```python
from build123d import *

# Parameters (mm, degrees)
SKETCH1_W           = 133.35
SKETCH1_H           = 38.1
BOSS_EXTRUDE1_DEPTH = 12.7
SKETCH2_R           = 3.175
CUT_EXTRUDE1_DEPTH  = 111.707422131
CAVITY1_DEPTH       = 12.7
CUT_EXTRUDE2_DEPTH  = 108.192417986
CUT_EXTRUDE4_DEPTH  = 108.192417986
CUT_EXTRUDE6_DEPTH  = 108.000606538
CUT_EXTRUDE7_DEPTH  = 105.814568341


# Read off the part's stored shape, not the designer's step: Cavity1
with BuildPart() as part:
    # Sketch1 → Boss-Extrude1 (new body)
    with BuildSketch(Plane.XY):
        with Locations((36.491047297, -7.135705236)):
            Rectangle(SKETCH1_W, SKETCH1_H)
    extrude(amount=BOSS_EXTRUDE1_DEPTH)

    # Sketch2 → Cut-Extrude1 (cut, through all)
    with BuildSketch(Plane(origin=(0, 11.914294764, 0), x_dir=(1, 0, 0), z_dir=(0, 1, 0))):
        with Locations(Location((-22.563952703, -6.35, 0), (0, 0, 270))):
            Circle(SKETCH2_R)
        with Locations(Location((25.188047297, -6.35, 0), (0, 0, 270))):
            Circle(SKETCH2_R)
    extrude(amount=-CUT_EXTRUDE1_DEPTH, mode=Mode.SUBTRACT)

    # Cavity1 outline → Cavity1 (cut)
    with BuildSketch(Plane.XY):
        with BuildLine():
            Line((96.096303093, 11.914294764), (94.056580093, 11.914294764))
            ThreePointArc((94.056580093, 11.914294764), (90.695637122, -2.438784083), (103.166047297, -10.299806924))
            Line((103.166047297, -10.299806924), (103.166047297, -9.052983376))
            ThreePointArc((103.166047297, -9.052983376), (91.591067883, -1.280306677), (96.096303093, 11.914294764))
        make_face()
    extrude(amount=CAVITY1_DEPTH, mode=Mode.SUBTRACT)

    # Sketch4 → Cut-Extrude2 (cut, through all)
    with BuildSketch(Plane(origin=(0, 0, 0), x_dir=(-1, 0, 0), z_dir=(0, 0, -1))):
        Polygon((-103.836015624, 12.337344095), (-103.707966328, -9.632256534), (-101.439664514, -9.485914481), (-98.220139359, -8.863960758), (-94.579880804, -6.924928563), (-91.031086031, -2.168811857), (-90.317668525, 2.879988954), (-91.085877767, 6.8566015), (-93.116460279, 9.831236447), (-96.207936138, 13.398323976), align=None)
    extrude(amount=-CUT_EXTRUDE2_DEPTH, mode=Mode.SUBTRACT)

    # Sketch9 → Cut-Extrude4 (cut, through all)
    with BuildSketch(Plane.XY.offset(12.7)):
        Polygon((-30.183952703, -13.474806924), (119.048045807, -13.474806924), (119.048045807, -32.591302601), (-30.183952703, -32.591302601), (-44.866857433, -32.591302601), (-44.866857433, 12.516766533), (-30.183952703, 12.516766533), align=None)
    extrude(amount=-CUT_EXTRUDE4_DEPTH, mode=Mode.SUBTRACT)

    # Sketch11 → Cut-Extrude6 (cut, through all)
    with BuildSketch(Plane(origin=(0, 11.914294764, 0), x_dir=(1, 0, 0), z_dir=(0, 1, 0))):
        with BuildLine():
            Line((-22.563952703, 0), (-30.183952703, 0))
            Line((-30.183952703, 0), (-30.183952703, -12.7))
            Line((-30.183952703, -12.7), (-22.563952703, -12.7))
            ThreePointArc((-22.563952703, -12.7), (-28.913952703, -6.35), (-22.563952703, 0))
        make_face()
    extrude(amount=-CUT_EXTRUDE6_DEPTH, mode=Mode.SUBTRACT)

    # Sketch12 → Cut-Extrude7 (cut, through all)
    with BuildSketch(Plane.XY):
        with BuildLine():
            Line((34.840047297, 8.739294764), (47.329311848, 8.739294764))
            ThreePointArc((47.329311848, 8.739294764), (63.205042995, 7.678873093), (78.798708551, 4.516448692))
            ThreePointArc((78.798708551, 4.516448692), (84.297585987, 1.423684462), (87.687974389, -3.896852177))
            Line((87.687974389, -3.896852177), (87.782466122, -4.180292862))
            ThreePointArc((87.782466122, -4.180292862), (87.135514906, -8.32519055), (83.381577499, -10.197802807))
            Line((83.381577499, -10.197802807), (46.450888554, -9.684330956))
            ThreePointArc((46.450888554, -9.684330956), (35.893420387, -5.181749435), (31.538047297, 5.437294764))
            ThreePointArc((31.538047297, 5.437294764), (32.505180706, 7.772161355), (34.840047297, 8.739294764))
        make_face()
        with BuildLine():
            Line((18.838047297, 5.437294764), (18.838047297, -6.997806924))
            ThreePointArc((18.838047297, -6.997806924), (17.870913889, -9.332673515), (15.536047297, -10.299806924))
            Line((15.536047297, -10.299806924), (-12.911952703, -10.299806924))
            ThreePointArc((-12.911952703, -10.299806924), (-15.246819294, -9.332673515), (-16.213952703, -6.997806924))
            Line((-16.213952703, -6.997806924), (-16.213952703, 5.437294764))
            ThreePointArc((-16.213952703, 5.437294764), (-15.246819294, 7.772161355), (-12.911952703, 8.739294764))
            Line((-12.911952703, 8.739294764), (15.536047297, 8.739294764))
            ThreePointArc((15.536047297, 8.739294764), (17.870913889, 7.772161355), (18.838047297, 5.437294764))
        make_face()
    extrude(amount=CUT_EXTRUDE7_DEPTH, mode=Mode.SUBTRACT)


solid = part.part
```
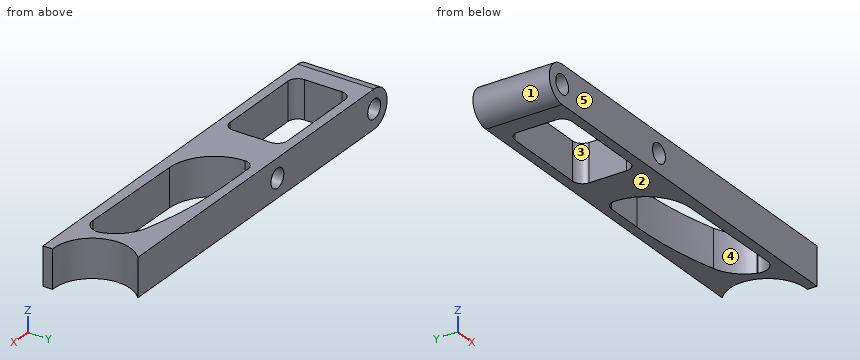
Geometry check sheet. Reference: the model listing, model coordinates, mm. Face numbers are marked on the shaded views. A direction names the side the tool comes from. Round coordinates to 2 decimals unless told otherwise and drop trailing zeros. Order: outer loops, then holes, each group sorted by start corner. A loop starts at its lowest first (then second) coordinate and runs counter-clockwise, first axis right, second up. Notation, with made-up numbers: (-11, 33.25) -> (-6, 33.25) arc R15 ccw to (-6, 50.25) -> close; hole circle Ø2 at (44.5, 1.25). An arc over 180 degrees is marked (long way). Return JSON: item names as keys, results as strings. Group by question number.
Q1. Tool access check on the marked faces 4 and 5. Record the directions out of +Z, -Z, +X, -X, +Y, -Y that give a thin tool (end or side, any length) a straight path to the whole face; none if there is none.
Q2. Section check A-A, the plane z = 6.35. Count the separate pieces of the cut face and the enclosed holes in it, plus the area to 3 significant figures.
Q3. Gauge pin test, flat ends, axial feed: pin 1 (6 mm diameter, centred on y = -4, z = 6, fed in from +X); pin 2 (3.5 mm diameter, centred on y = -2.5, z = 3.5, fed in from -X); pin 3 (2 mm diameter, centred on y = 5.5, z = 6, fed in from +X). Record the tip position at first contact, or that the pin passes through.
Q4. Section check C-C, the plane x = 33. Record the boundary of the cut face in (y, z), plus the area to 3 significant figures.
Q5. Material ranges on probe 1 along Y at (x, z) = (0, 1); probe 2 along X at (y, z) = (3.5, 11.25); probe 3 along Y at (x, z) = (82, 2.25), recorded low to high. Write a range as from..to.
Q6. Release check for a two-part mould opening along X. For the marked faces 1, 2 and 3 record: released by +X, released by -X, zero draft, split by the parting line, or undercut.
Q7. Section check D-D, the plane x = 84.5. Record the boundary of the cut face in (y, z), plus the area to 3 significant figures.
Q8. Section check B-B, the plane y = 2. Record the boundary of the cut face in (x, z) (3 decimals), plus the area to 4 significant figures.
Numbers:
{
 "1": {"face 4": "+Z, -Z", "face 5": "+Z, -Z, +X, -X, -Y"},
 "2": {"separate pieces": "3", "enclosed holes": "2", "area": "1,240 mm^2"},
 "3": {"pin 1": "x = 93.88", "pin 2": "x = -28.82", "pin 3": "x = 90.43"},
 "4": {"outline": "(-13.47, 0) -> (-1.05, 0) -> (-1.05, 12.7) -> (-13.47, 12.7) -> close; (8.18, 0) -> (11.91, 0) -> (11.91, 12.7) -> (8.18, 12.7) -> close", "area": "205 mm^2"},
 "5": {"probe 1": "-13.47..-10.3, 8.74..11.91", "probe 2": "-26.6..-16.21, 18.84..31.66, 81.39..89.8", "probe 3": "-13.47..-10.18, 3.16..11.91"},
 "6": {"face 1": "released by -X", "face 2": "zero draft", "face 3": "undercut"},
 "7": {"outline": "(-13.47, 0) -> (-10.07, 0) -> (-10.07, 12.7) -> (-13.47, 12.7) -> close; (1.23, 0) -> (11.91, 0) -> (11.91, 12.7) -> (1.23, 12.7) -> close", "area": "179 mm^2"},
 "8": {"outline": "(-22.564, 0) -> (-16.214, 0) -> (-16.214, 12.7) -> (-22.564, 12.7) arc R6.35 ccw to start; (18.838, 0) -> (31.934, 0) -> (31.934, 12.7) -> (18.838, 12.7) -> close; (83.646, 0) -> (89.752, 0) -> (89.752, 12.7) -> (83.646, 12.7) -> close; hole circle Ø6.35 at (-22.564, 6.35); hole circle Ø6.35 at (25.188, 6.35)", "area": "324.5 mm^2"}
}
